from build123d import *

# Parameters (mm, degrees)
RESSALTO_EXTRUS_O2_DEPTH = 6
RESSALTO_EXTRUS_O3_DEPTH = 6
CORTE_EXTRUS_O1_DEPTH    = 303.732253462


with BuildPart() as part:
    # Esboço1 → Ressalto-extrusão2 (new body)
    with BuildSketch(Plane.XY):
        with BuildLine():
            Line((-199.999999999, 0), (199.999999999, 0))
            ThreePointArc((199.999999999, 0), (202.565835097, -15.811388301), (209.999999999, -30))
            Line((209.999999999, -30), (289.999999999, -30))
            ThreePointArc((289.999999999, -30), (299.999014124, 0.31398499), (289.62007067, 30.5))
            ThreePointArc((289.62007067, 30.5), (297.818976076, 75.60635228), (265.815415017, 108.432822474))
            Line((265.815415017, 108.432822474), (246.403986634, 35.988385502))
            ThreePointArc((246.403986634, 35.988385502), (242.72975202, 33.867065158), (240.608431676, 37.541299773))
            Line((240.608431676, 37.541299773), (260.019860059, 109.985736744))
            ThreePointArc((260.019860059, 109.985736744), (218.38507475, 99.736242739), (199.999999999, 61))
            Line((199.999999999, 61), (140, 61))
            Line((140, 61), (150.784643454, 58.387579086))
            Line((150.784643454, 58.387579086), (139.047219324, 52.742194858))
            Line((139.047219324, 52.742194858), (160.085396074, 40.245061921))
            Line((160.085396074, 40.245061921), (137.597498913, 43.437533109))
            Line((137.597498913, 43.437533109), (153.154101004, 34.194272541))
            Line((153.154101004, 34.194272541), (138.26257587, 30.30469508))
            Line((138.26257587, 30.30469508), (144.152507453, 26))
            Line((144.152507453, 26), (149.999999999, 26))
            ThreePointArc((149.999999999, 26), (152.999999999, 23), (149.999999999, 20))
            Line((149.999999999, 20), (-149.999999999, 20))
            ThreePointArc((-149.999999999, 20), (-152.999999999, 23), (-149.999999999, 26))
            Line((-149.999999999, 26), (-144.152507453, 26))
            Line((-144.152507453, 26), (-138.26257587, 30.30469508))
            Line((-138.26257587, 30.30469508), (-153.154101004, 34.194272541))
            Line((-153.154101004, 34.194272541), (-137.597498913, 43.437533109))
            Line((-137.597498913, 43.437533109), (-160.085396074, 40.245061921))
            Line((-160.085396074, 40.245061921), (-139.047219324, 52.742194858))
            Line((-139.047219324, 52.742194858), (-150.784643454, 58.387579086))
            Line((-150.784643454, 58.387579086), (-140, 61))
            Line((-140, 61), (-199.999999999, 61))
            ThreePointArc((-199.999999999, 61), (-218.38507475, 99.736242739), (-260.019860059, 109.985736744))
            Line((-260.019860059, 109.985736744), (-240.608431676, 37.541299773))
            ThreePointArc((-240.608431676, 37.541299773), (-242.72975202, 33.867065158), (-246.403986634, 35.988385502))
            Line((-246.403986634, 35.988385502), (-265.815415017, 108.432822474))
            ThreePointArc((-265.815415017, 108.432822474), (-297.818976076, 75.60635228), (-289.62007067, 30.5))
            ThreePointArc((-289.62007067, 30.5), (-299.999014124, 0.31398499), (-289.999999999, -30))
            Line((-289.999999999, -30), (-209.999999999, -30))
            ThreePointArc((-209.999999999, -30), (-202.565835097, -15.811388301), (-199.999999999, 0))
        make_face()
    extrude(amount=RESSALTO_EXTRUS_O2_DEPTH)


with BuildPart() as body_2:
    # Esboço4 → Ressalto-extrusão3 (new body)
    with BuildSketch(Plane(origin=(215.105397993, -57.63731768, 0), x_dir=(0, 0, -1), z_dir=(0.9659258262890679, -0.25881904510252246, 0))):
        with BuildLine():
            Line((246.999999999, 62.536155533), (246.999999999, 123.536155533))
            Line((246.999999999, 123.536155533), (47, 123.536155533))
            ThreePointArc((47, 123.536155533), (32.355339059, 158.891494592), (-3, 173.536155533))
            ThreePointArc((-3, 173.536155533), (-47.860896112, 145.615557699), (-42.620070671, 93.036155533))
            ThreePointArc((-42.620070671, 93.036155533), (-52.987511897, 61.418723482), (-41.217566642, 30.296155533))
            Line((-41.217566642, 30.296155533), (35.217566642, 30.296155533))
            ThreePointArc((35.217566642, 30.296155533), (43.96210351, 45.373380875), (47, 62.536155533))
            Line((47, 62.536155533), (246.999999999, 62.536155533))
        make_face()
    extrude(amount=RESSALTO_EXTRUS_O3_DEPTH)

    # Combinar1: cut part
    add(part.part, mode=Mode.SUBTRACT)

    # Esboço6 → Corte-extrusão1 (cut, through all)
    with BuildSketch(Plane(origin=(220.900952951, -59.190231951, 0), x_dir=(0, 0, -1), z_dir=(0.9659258262890679, -0.2588190451025225, 0))):
        with BuildLine():
            Line((-6, 98.536155533), (-6, 92.597624289))
            Line((-6, 92.597624289), (0, 92.597624289))
            Line((0, 92.597624289), (0, 98.536155533))
            ThreePointArc((0, 98.536155533), (-3, 101.536155533), (-6, 98.536155533))
        make_face()
    extrude(amount=-CORTE_EXTRUS_O1_DEPTH, mode=Mode.SUBTRACT)

    # Espelhar2: body 2 across plane


with BuildPart() as body_2_1:
    add(body_2.part)
    add(body_2.part.mirror(Plane(origin=(237.086501011, 1.215055756, -246.999999999), x_dir=(1, 0, 0), z_dir=(0, 0, 1))))


solid = body_2_1.part
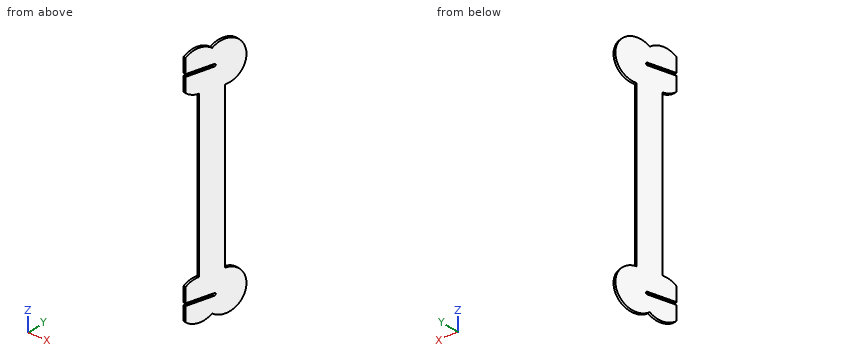
Part model, mm, in its own coordinate system. Give positions to 0.01 mm unless a question says otherwise; leave off trailing zeros. Order: outer loops, then holes, each group sorted by start corner. A loop starts at its lowest first (then second) coordinate and runs counter-clockwise, first axis right, second up. Notation, with made-up numbers: (-36, 75.25) - (9, 75.25) arc R19 ccw to (9, 108.25) - close; hole circle Ø10 at (-3.5, 75.25). An arc over 180 degrees is marked (long way). Use a Markdown table: item, result.
1) Saw through at A-A on z = -136. List the corners of the cut face in (x, y).
Checked values:
| item | result |
|---|---|
| outline | (231.29, 2.77) - (237.09, 1.22) - (252.87, 60.14) - (247.08, 61.69) - close |
2) Flat gauge pins, fed straight in: P1, Ø6, axis at y = -2, z = -483, coming from the +X side; P2, Ø10, axis at x = 246.5, z = -127, coming from the +Y side; P3, Ø11.5, axis at x = 233.5, y = -11.5, coming from the -Z side. Where does each tip first touch, or does it go through?
Checked values:
| item | result |
|---|---|
| P1 | x = 237.03 |
| P2 | y = 61.69 |
| P3 | z = -546.44 |
3) Probe L1, parallel to Z at x = 234, y = 6.5; L2, parallel to Z at x = 249.5, y = 65; L3, parallel to X at y = 50, z = 5.5. List the from-to ranges inside material, lowest first. Write a range as from..to.
Checked values:
| item | result |
|---|---|
| L1 | -546.81..-500, -494..0, 6..52.81 |
| L2 | -546.85..-447.15, -46.85..52.85 |
| L3 | 243.95..250.16 |
4) Saw through at D-D on z = -26. List the corners of the cut face in (x, y), plus the area to 3 significant figures.
Checked values:
| item | result |
|---|---|
| outline | (222.95, -28.37) - (228.74, -29.93) - (263.42, 99.48) - (257.62, 101.03) - close |
| area | 804 mm² |
5) Saw through at B-B on y = 23. Count the separate pieces of the cut face and the enclosed holes in it, plus the area to 3 significant figures.
Checked values:
| item | result |
|---|---|
| separate pieces | 3 |
| enclosed holes | 0 |
| area | 3,590 mm² |
